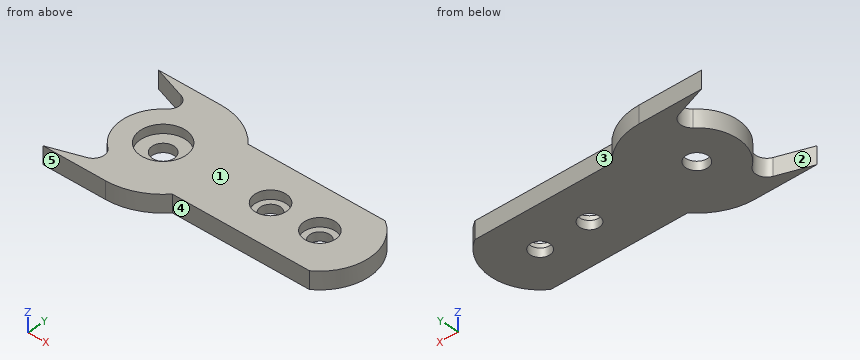
```python
from build123d import *

# Parameters (mm, degrees)
SKETCH1_R           = 10
BOSS_EXTRUDE1_DEPTH = 7.9375
FILLET1_R           = 10
SKETCH2_R           = 14.2875
CUT_EXTRUDE1_DEPTH  = 8
SKETCH3_R           = 9
CUT_EXTRUDE2_DEPTH  = 198.022009439
SKETCH4_R           = 20.6375
CUT_EXTRUDE3_DEPTH  = 7.9375


with BuildPart() as part:
    # Sketch1 → Boss-Extrude1 (new, symmetric)
    with BuildSketch(Plane.XY):
        with BuildLine():
            Line((-57, -57), (0, -37.5))
            ThreePointArc((0, -37.5), (-37.5, 0), (0, 37.5))
            Line((0, 37.5), (-57, 57))
            Line((-57, 57), (0, 57))
            ThreePointArc((0, 57), (23.574350468, 51.896531676), (42.927264064, 37.5))
            Line((42.927264064, 37.5), (167.927264064, 37.5))
            ThreePointArc((167.927264064, 37.5), (187.927264064, 0), (167.927264064, -37.5))
            Line((167.927264064, -37.5), (42.927264064, -37.5))
            ThreePointArc((42.927264064, -37.5), (23.574350468, -51.896531676), (0, -57))
            Line((0, -57), (-57, -57))
        make_face()
        Circle(SKETCH1_R, mode=Mode.SUBTRACT)
    extrude(amount=BOSS_EXTRUDE1_DEPTH, both=True)

    # Fillet1
    fillet1_edges = [part.edges().sort_by_distance(p)[0] for p in [
        (0, -37.5, 0),
        (0, 37.5, 0),
    ]]
    fillet(fillet1_edges, radius=FILLET1_R)

    # Sketch2 → Cut-Extrude1 (cut)
    with BuildSketch(Plane.XY.offset(7.9375)):
        with Locations((142.927264064, 0)):
            Circle(SKETCH2_R)
        with Locations((97.927264064, 0)):
            Circle(SKETCH2_R)
    extrude(amount=-CUT_EXTRUDE1_DEPTH, mode=Mode.SUBTRACT)

    # Sketch3 → Cut-Extrude2 (cut, through all)
    with BuildSketch(Plane.XY.offset(7.9375)):
        with Locations((97.927264064, 0)):
            Circle(SKETCH3_R)
        with Locations((142.927264064, 0)):
            Circle(SKETCH3_R)
    extrude(amount=-CUT_EXTRUDE2_DEPTH, mode=Mode.SUBTRACT)

    # Sketch4 → Cut-Extrude3 (cut)
    with BuildSketch(Plane.XY.offset(7.9375)):
        Circle(SKETCH4_R)
    extrude(amount=-CUT_EXTRUDE3_DEPTH, mode=Mode.SUBTRACT)


solid = part.part
```
Input: part model. Units: mm. Frame: model coordinates. Face numbers are marked on the shaded views. A direction names the side the tool comes from. Round coordinates to 2 decimals unless told otherwise and drop trailing zeros. Loops run counter-clockwise (first coordinate to the right, second up) from the corner with the lowest first, then second, coordinate; pieces in that order, holes last. Notation, with made-up numbers: (16.5, -25.5) - (26.5, -25.5) arc R22 cw to (26.5, -17.5) - close; hole circle Ø1 at (-21.75, 29.5). An arc over 180 degrees is marked (long way). One line per item, written item: value. Start each with the question number.
(1) Section A-A, the plane y = 0. Return loops of the section in (x, z), plus the area to 3 significant figures.
(2) Section B-B, the plane z = -5. Return loops of the section in (x, y), plus the area to 3 significant figures.
(3) Access query for the marked faces 1, 2, 3, 4 and 5. Directions: +Z, -Z, +X, -X, +Y, -Y. A direction counts if a zero-diameter tool reaches every point of the face in a straight line with its end or side. Return the directions, or none.
(4) Contact query for flat-ended pins moving along their axis: P1, Ø20.5, axis at x = 142.93, y = 0, coming from the +Z side; P2, Ø23, axis at x = 0, y = 0, coming from the +Z side; P3, Ø4, axis at y = 21, z = -5.5, coming from the +X side. Output: stop coordinate, or through.
(5) Section C-C, the plane x = 144.5. Return loops of the section in (y, z).
(6) Ray query, line 1 (Y direction, x = 97, z = 1.5); line 2 (X direction, y = 14.5, z = 2.5); line 3 (Y direction, x = 100.5, z = 5.25). Return the intervals inside material, ascending. Write a range as [from, to].
(7) Section D-D, the plane x = 91.5. Return loops of the section in (y, z).
Results below:
1. outline: (-37.5, -7.94) - (-10, -7.94) - (-10, 0) - (-20.64, 0) - (-20.64, 7.94) - (-37.5, 7.94) - close; (10, -7.94) - (88.93, -7.94) - (88.93, -0.06) - (83.64, -0.06) - (83.64, 7.94) - (20.64, 7.94) - (20.64, 0) - (10, 0) - close; (106.93, -7.94) - (133.93, -7.94) - (133.93, -0.06) - (128.64, -0.06) - (128.64, 7.94) - (112.21, 7.94) - (112.21, -0.06) - (106.93, -0.06) - close; (151.93, -7.94) - (187.93, -7.94) - (187.93, 7.94) - (157.21, 7.94) - (157.21, -0.06) - (151.93, -0.06) - close
1. area: 2,350 mm^2
2. outline: (-57, -57) - (0, -57) arc R57 ccw to (42.93, -37.5) - (167.93, -37.5) arc R45.16 ccw to (167.93, 37.5) - (42.93, 37.5) arc R57 ccw to (0, 57) - (-57, 57) - (-26.44, 46.55) arc R10 cw to (-23.43, 29.28) arc R37.5 ccw to (-23.43, -29.28) arc R10 cw to (-26.44, -46.55) - close; hole circle Ø20 at (0, 0); hole circle Ø18 at (97.93, 0); hole circle Ø18 at (142.93, 0)
2. area: 17,500 mm^2
3. face 1: +Z, +X, -X, +Y, -Y
3. face 2: +Z, -Z, -X
3. face 3: +Z, -Z, +X, +Y
3. face 4: +Z, -Z, +X, -Y
3. face 5: +Z, -Z, +X, -X, -Y
4. P1: z = -0.06
4. P2: z = 0
4. P3: x = 183.74
5. outline: (-37.5, -7.94) - (-8.86, -7.94) - (-8.86, -0.06) - (-14.2, -0.06) - (-14.2, 7.94) - (-37.5, 7.94) - close; (8.86, -7.94) - (37.5, -7.94) - (37.5, 7.94) - (14.2, 7.94) - (14.2, -0.06) - (8.86, -0.06) - close
6. line 1: [-37.5, -14.26], [14.26, 37.5]
6. line 2: [-34.58, -14.69], [14.69, 185.54]
6. line 3: [-37.5, -14.05], [14.05, 37.5]
7. outline: (-37.5, -7.94) - (-6.3, -7.94) - (-6.3, -0.06) - (-12.76, -0.06) - (-12.76, 7.94) - (-37.5, 7.94) - close; (6.3, -7.94) - (37.5, -7.94) - (37.5, 7.94) - (12.76, 7.94) - (12.76, -0.06) - (6.3, -0.06) - close
